from build123d import *

# Parameters (mm, degrees)
U_SHAPE_DEPTH        = 100
SKETCH8_R            = 13.870670921
INNER_HOLE_DEPTH     = 126.918394305
THICKNESS_T          = -20
FILLET_2_R           = 12
TONGUE_DEPTH         = 20
SKETCH9_R            = 13.219756801
MOUNTING_HOLES_DEPTH = 223.42572915


with BuildPart() as part:
    # Sketch4 → "U" shape (new body)
    with BuildSketch(Plane.XY):
        with BuildLine():
            Line((-45.388843922, 0), (-45.388843922, -61.60596458))
            Line((-45.388843922, -61.60596458), (45.388843922, -61.60596458))
            Line((45.388843922, -61.60596458), (45.388843922, 0))
            ThreePointArc((45.388843922, 0), (0, 45.388843922), (-45.388843922, 0))
        make_face()
    extrude(amount=U_SHAPE_DEPTH)

    # Sketch8 → Inner Hole (cut, through all)
    with BuildSketch(Plane.XY.offset(100)):
        with Locations((38.923783738, 0.23491683)):
            Circle(SKETCH8_R)
    extrude(amount=-INNER_HOLE_DEPTH, mode=Mode.SUBTRACT)

    # Thickness
    thickness_openings = [part.faces().sort_by_distance(p)[0] for p in [
        (45.388843922, -36.821453076, 50),
        (-45.388843922, -30.80298229, 50),
        (-6.761547736, 44.882386576, 50),
    ]]
    offset(amount=THICKNESS_T, openings=thickness_openings, kind=Kind.INTERSECTION)

    # Fillet 2
    fillet_2_edges = [part.edges().sort_by_distance(p)[0] for p in [
        (0, -61.60596458, 100),
        (0, -61.60596458, 0),
    ]]
    fillet(fillet_2_edges, radius=FILLET_2_R)

    # Sketch7 → Tongue (add)
    with BuildSketch(Plane.XZ.offset(64.60596458)):
        with BuildLine():
            Line((24.518796564, 26.143873614), (154.843931452, 5.821988173))
            ThreePointArc((154.843931452, 5.821988173), (167.031484247, 13.741465613), (160.484216098, 26.717899862))
            Line((160.484216098, 26.717899862), (37.634315602, 74.733748908))
            Line((37.634315602, 74.733748908), (24.518796564, 26.143873614))
        make_face()
    extrude(amount=-TONGUE_DEPTH)

    # Sketch9 → Mounting Holes (cut, through all)
    with BuildSketch(Plane.XZ.offset(61.60596458)):
        with Locations((73.545474364, 50)):
            Circle(SKETCH9_R)
        with Locations((125.389042853, 44.726843721)):
            Circle(SKETCH9_R)
    extrude(amount=-MOUNTING_HOLES_DEPTH, mode=Mode.SUBTRACT)


solid = part.part
Build history of the part. All positions in model axes, mm. A direction names the side the tool comes from. Give positions to 0.01 mm unless a question says otherwise; leave off trailing zeros. Order: outer loops, then holes, each group sorted by start corner. A loop starts at its lowest first (then second) coordinate and runs counter-clockwise, first axis right, second up. Notation, with made-up numbers: M 69,23 L 97,23 A28 cw 97,45 Z; hole C 43,6 d11. An arc over 180 degrees is marked long. Put each result on its own line as item: value.
Item 1: Slice it at B-B, the plane x = 20. Write the cut outline in (y, z), plus the area to 3 significant figures.
From the geometry:
outline: M -61.61,12 A12 ccw -49.61,0 L 40.74,0 L 40.74,20 L 28.33,20 L 28.33,80 L 40.74,80 L 40.74,100 L -49.61,100 A12 ccw -61.61,88 Z; hole M -41.61,20 L -27.86,20 L -27.86,80 L -41.61,80 Z
area: 8,600 mm2
Item 2: 3-axis set-ups, long thin cutter, end or side, ignore diameter. For faces 4 (the flat face through (73, -61.606, 50)), 5 (the flat face through (106, -44.606, 32)), 6 (the flat face through (31.17, -63.13, 50.78)), 7 (the cylindrical face through (25.07, -0.48, 50.7)): which of +Z, -Z, +X, -X, +Y, -Y reach the whole face in a straight line?
From the geometry:
face 4: +Y
face 5: +Z, -Z, +X, +Y
face 6: +Z, -X, -Y
face 7: +Z, -Z
Item 3: Slice it at D-D, the plane x = -11.5. Write the cut outline in (y, z), plus the area to 3 significant figures.
From the geometry:
outline: M -61.61,12 A12 ccw -49.61,0 L 43.91,0 L 43.91,20 L -41.61,20 L -41.61,80 L 43.91,80 L 43.91,100 L -49.61,100 A12 ccw -61.61,88 Z
area: 5,360 mm2
Item 4: Two-plate mould, pull along Y, no slides. Class faces 1 (the flat face through (-1, -41.606, 50)), 2 (the flat face through (-45.389, -44, 49)), 3 (the flat face through (121, -61.606, 37)): +Y half, -Y half, draft (parallel to the pull), parting line (faces both ways), or undercut.
From the geometry:
face 1: undercut
face 2: draft
face 3: +Y half
Item 5: Probe line 1 (Z direction, x = 5, y = 14); line 2 (Y direction, x = 36, z = 72); line 3 (Y direction, x = 154, z = 23). List the from-to ranges inside material, lowest first. Write a range as [from, to].
From the geometry:
line 1: z = [0, 20], [80, 100]
line 2: y = [-61.61, -41.61], [-33.51, -13.32], [13.79, 27.64]
line 3: y = [-64.61, -44.61]
Item 6: Slice it at C-C, the plane y = 21. Write the cut outline in (x, z), plus the area to 3 significant figures.
From the geometry:
outline: M -40.24,0 L 40.24,0 L 40.24,100 L -40.24,100 L -40.24,80 L 12.16,80 L 12.16,20 L -40.24,20 Z
area: 4,900 mm2
Item 7: Slice it at A-A, the plane z = 52. Write the cut outline in (x, y), plus the area to 3 significant figures.
From the geometry:
outline: M -45.39,-61.61 L 31.5,-61.61 L 31.5,-64.61 L 95.8,-64.61 L 95.8,-44.61 L 86.61,-44.61 L 86.61,-61.61 L 60.48,-61.61 L 60.48,-44.61 L 45.39,-44.61 L 45.39,-41.61 L -45.39,-41.61 Z; M 30.99,33.16 A33.87 ccw 45.39,-33.01 L 45.39,-12.04 A13.87 cw long 43.37,13.37 A45.39 ccw Z
area: 4,030 mm2
Item 8: Flat gauge pins, fed straight in: pin 1 Ø18 at (x, z) = (-21, 57.5) entering from +Y; pin 2 Ø1.5 at (y, z) = (-39.5, 57) entering from -X; pin 3 Ø5 at (y, z) = (27, 78) entering from +X; pin 4 Ø4 at (x, z) = (120.5, 41.5) entering from +Y. Where does each tip first touch, or does it go through?
From the geometry:
pin 1: stops at y = -41.61
pin 2: passes through
pin 3: stops at x = 38.21
pin 4: stops at y = -61.61
